Verification items for the finished model (mm, model axes). Coordinates: 2 decimals unless noted, no trailing zeros. Order: outer loops, then holes, each group sorted by start corner. A loop starts at its lowest first (then second) coordinate and runs counter-clockwise, first axis right, second up. Notation, with made-up numbers: M 20,35.5 L 55,35.5 A29 cw 55,64.5 Z; hole C 2,-20 d11. An arc over 180 degrees is marked long. Write item = value, one per line.
```python
from build123d import *

# Parameters (mm, degrees)
SKETCH_1_W          = 140
SKETCH_1_H          = 100
EXTRUDE_1_DEPTH     = 1.6
SKETCH_2_R          = 1.6
CUT_EXTRUDE_1_DEPTH = 87.038131082


with BuildPart() as part:
    # Эскиз1 → Бобышка-Вытянуть1 (new body)
    with BuildSketch(Plane.XY):
        Rectangle(SKETCH_1_W, SKETCH_1_H)
    extrude(amount=EXTRUDE_1_DEPTH)

    # Эскиз2 → Вырез-Вытянуть1 (cut, through all)
    with BuildSketch(Plane.XY.offset(1.6)):
        with Locations((-65.9, 45.75)):
            Circle(SKETCH_2_R)
        with Locations(Location((65.9, 45.75, 0), (0, 0, 180))):
            Circle(SKETCH_2_R)
        with Locations((65.9, -45.75)):
            Circle(SKETCH_2_R)
        with Locations(Location((-65.9, -45.75, 0), (0, 0, 180))):
            Circle(SKETCH_2_R)
        with Locations(Location((55.9, 45.75, 0), (0, 0, 180))):
            Circle(SKETCH_2_R)
        with Locations((55.9, -45.75)):
            Circle(SKETCH_2_R)
    extrude(amount=-CUT_EXTRUDE_1_DEPTH, mode=Mode.SUBTRACT)


solid = part.part
```
Item 1: Sectioned sample at A-A, the plane x = 65.9. Enter the section's corners in (y, z).
Report:
outline = M -50,0 L -47.35,0 L -47.35,1.6 L -50,1.6 Z; M -44.15,0 L 44.15,0 L 44.15,1.6 L -44.15,1.6 Z; M 47.35,0 L 50,0 L 50,1.6 L 47.35,1.6 Z
Item 2: Sectioned sample at B-B, the plane y = 45.75. Enter the section's corners in (x, z).
Report:
outline = M -70,0 L -67.5,0 L -67.5,1.6 L -70,1.6 Z; M -64.3,0 L 54.3,0 L 54.3,1.6 L -64.3,1.6 Z; M 57.5,0 L 64.3,0 L 64.3,1.6 L 57.5,1.6 Z; M 67.5,0 L 70,0 L 70,1.6 L 67.5,1.6 Z
Item 3: Gauge pin test, flat ends, axial feed: pin 1 (4 mm diameter, centred on x = -65.9, y = -45.75, fed in from +Z); pin 2 (3 mm diameter, centred on x = 55.9, y = 45.75, fed in from +Z). Record the tip position at first contact, or that the pin passes through.
Report:
pin_1 = 1.6
pin_2 = through
Item 4: Scan lines: L1, parallel to Y at x = -65.9, z = 0.85; L2, parallel to X at y = 45.5, z = 0.35; L3, parallel to Y at x = 57, z = 0.8. Record each from-to range of solid material in increasing order. Write a range as from..to.
Report:
L1 = -50..-47.35, -44.15..44.15, 47.35..50
L2 = -70..-67.48, -64.32..54.32, 57.48..64.32, 67.48..70
L3 = -50..-46.91, -44.59..44.59, 46.91..50
Item 5: Release check for a two-part mould opening along X. For faces 1 (the flat face through (-1, 1, 1.6)), 2 (the cylindrical face through (64.374, 45.269, 0.811)) record: pulls with the +X half, pulls with the -X half, needs draft (parallel to the pull), parting line crosses it, or undercut.
Report:
face_1 = needs draft
face_2 = undercut
